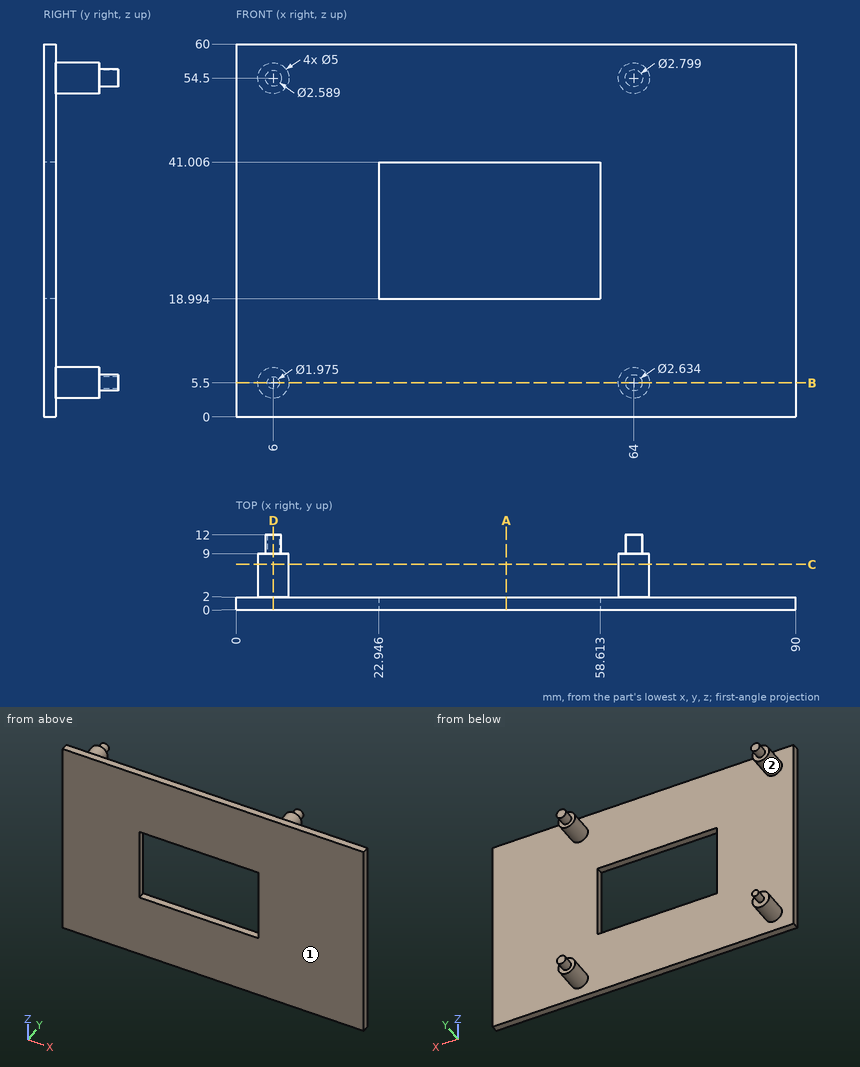
Study the drawing (mm; zero at the part's minimum x, y, z) and answer. Coordinates: 2 decimals unless noted, no trailing zeros. Write each loop counter-clockwise with the first axis right and the second up, starting at its lowest first coordinate (ties: lowest second). Pieces come first, ordered by that corner, then holes. Notation, with made-up numbers: (-28.5, 69.5) - (-13.5, 69.5) arc R25 ccw to (-13.5, 96.5) - close; hole circle Ø4 at (57.5, 83.5). An arc over 180 degrees is marked (long way). Put each result on its own line as item: value.
1. The part is cut by section A-A on x = 43.5. Give the vertices of the cut face in (y, z) (1 decimal).
Answer sheet:
outline: (0, 0) - (2, 0) - (2, 19) - (0, 19) - close; (0, 41) - (2, 41) - (2, 60) - (0, 60) - close
2. Flat-ended cylindrical pins translate along their axes: pin 1 Ø18 at (x, z) = (52.5, 30.5) entering from +Y; pin 2 Ø3 at (y, z) = (4, 52) entering from +X. Find the tip coordinate at first contact, or state that the pin passes through.
Answer sheet:
pin 1: stops at y = 2
pin 2: stops at x = 66.29
3. The part is cut by section B-B on z = 5.5. Give the vertices of the cut face in (x, y), plus the area to 3 significant figures.
Answer sheet:
outline: (0, 0) - (90, 0) - (90, 2) - (66.5, 2) - (66.5, 9) - (65.32, 9) - (65.32, 12) - (62.68, 12) - (62.68, 9) - (61.5, 9) - (61.5, 2) - (8.5, 2) - (8.5, 9) - (6.99, 9) - (6.99, 12) - (5.01, 12) - (5.01, 9) - (3.5, 9) - (3.5, 2) - (0, 2) - close
area: 264 mm^2
4. Determine the mould class of the marked faces 1 and 2 for opening direction X: pulls with the +X half, pulls with the -X half, needs draft (parallel to the pull), parting line crosses it, or undercut.
Answer sheet:
face 1: needs draft
face 2: undercut
5. The part is cut by section C-C on y = 7.25. Give the vertices of the cut face in (x, z).
Answer sheet:
outline: circle Ø5 at (6, 5.5); circle Ø5 at (6, 54.5); circle Ø5 at (64, 5.5); circle Ø5 at (64, 54.5)
6. Find the intervals of material crossed by line 1 along Z through (x, y) = (35, 1.5) (1 decimal); line 2 along Y through (x, z) = (7, 52); line 3 along X through (y, z) = (3.25, 5), in increasing order. Write a range as from..to.
Answer sheet:
line 1: z = 0..19, 41..60
line 2: y = 0..2
line 3: x = 3.55..8.45, 61.55..66.45
7. The part is cut by section D-D on x = 6. Give the vertices of the cut face in (y, z) (1 decimal).
Answer sheet:
outline: (0, 0) - (2, 0) - (2, 3) - (9, 3) - (9, 4.5) - (12, 4.5) - (12, 6.5) - (9, 6.5) - (9, 8) - (2, 8) - (2, 52) - (9, 52) - (9, 53.2) - (12, 53.2) - (12, 55.8) - (9, 55.8) - (9, 57) - (2, 57) - (2, 60) - (0, 60) - close
